Input: part model. Units: mm. Frame: model coordinates. Face numbers are marked on the shaded views. Coordinates: 2 decimals unless noted, no trailing zeros. Loops run counter-clockwise (first coordinate to the right, second up) from the corner with the lowest first, then second, coordinate; pieces in that order, holes last. Notation, with made-up numbers: (-1, -3) - (14, -3) arc R21 ccw to (14, 2) - close; hole circle Ø7 at (-7, -2.75). An arc over 180 degrees is marked (long way). Use a Markdown table: item, result. Add a question column.
1. Section query A-A on y = 0. Return the cut outline in (x, z).
2. Section query B-B on z = 12. Return the cut outline in (x, y), then the cut area to 3 significant figures.
3. Ray query, L1, parallel to X at y = 0, z = 1.2; L2, parallel to X at y = 2.75, z = 4.75. Return the intervals inside material, ascending. Write a range as [from, to].
4. Draft query along Z for the marked faces 1, 2, 3 and 4. Return one class per face: released by +Z, released by -Z, zero draft, split by the parting line, or undercut.
5. Section query D-D on x = 1. Return the cut outline in (y, z), then the cut area to 3 significant figures.
6. Section query C-C on y = 5.25. Return the cut outline in (x, z), then the cut area to 3 significant figures.
7. Contact query for flat-ended pins moving along their axis: P1, Ø5, axis at y = 0, z = 12, coming from the +X side; P2, Ø5.5, axis at y = 0, z = 10.46, coming from the -X side; P3, Ø3.5, axis at x = 9, y = -1.5, coming from the +Z side; P4, Ø2, axis at x = 11.5, z = 3, coming from the -Y side. Output: stop coordinate, or through.
```python
from build123d import *

# Parameters (mm, degrees)
PAD_DEPTH       = 6.35
SKETCH001_R     = 1.778
POCKET_DEPTH    = 14.2758
SKETCH002_R     = 1.778
POCKET001_DEPTH = 14.2758


with BuildPart() as part:
    # Sketch → Pad (new body, symmetric)
    with BuildSketch(Plane.XZ):
        with BuildLine():
            Line((0, 14.2748), (0, 1.27))
            ThreePointArc((0, 1.27), (0.371974, 0.371974), (1.27, 0))
            Line((1.27, 0), (14.2748, 0))
            Line((14.2748, 0), (14.2748, 1.5748))
            Line((14.2748, 1.5748), (2.8448, 1.5748))
            ThreePointArc((1.5748, 2.8448), (1.946774, 1.946774), (2.8448, 1.5748))
            Line((1.5748, 2.8448), (1.5748, 14.2748))
            Line((1.5748, 14.2748), (0, 14.2748))
        make_face()
    extrude(amount=PAD_DEPTH, both=True)

    # Sketch001 → Pocket (cut, through all)
    with BuildSketch(Plane.XY):
        with Locations((10.4648, 0)):
            Circle(SKETCH001_R)
    extrude(amount=POCKET_DEPTH, mode=Mode.SUBTRACT)

    # Sketch002 → Pocket001 (cut, through all)
    with BuildSketch(Plane.YZ):
        with Locations((0, 10.4648)):
            Circle(SKETCH002_R)
    extrude(amount=POCKET001_DEPTH, mode=Mode.SUBTRACT)


solid = part.part
```
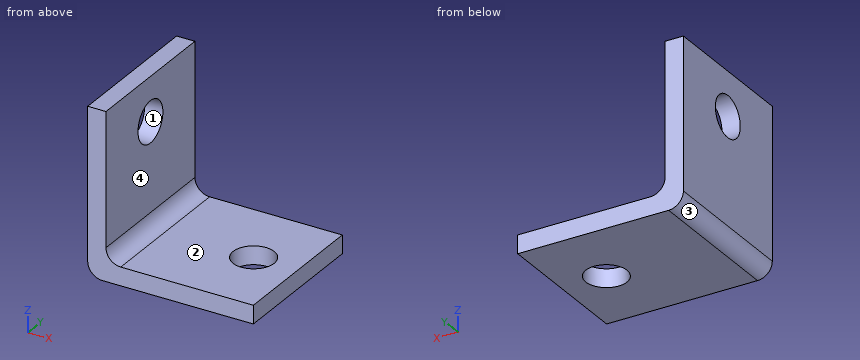
Resolved:
| question | item | result |
|---|---|---|
| 1 | outline | (0, 1.27) arc R1.27 ccw to (1.27, 0) - (8.69, 0) - (8.69, 1.57) - (2.84, 1.57) arc R1.27 cw to (1.57, 2.84) - (1.57, 8.69) - (0, 8.69) - close; (0, 12.24) - (1.57, 12.24) - (1.57, 14.27) - (0, 14.27) - close; (12.24, 0) - (14.27, 0) - (14.27, 1.57) - (12.24, 1.57) - close |
| 2 | outline | (0, -6.35) - (1.57, -6.35) - (1.57, -0.9) - (0, -0.9) - close; (0, 0.9) - (1.57, 0.9) - (1.57, 6.35) - (0, 6.35) - close |
| 2 | area | 17.2 mm² |
| 3 | L1 | [0, 8.69], [12.24, 14.27] |
| 3 | L2 | [0, 1.57] |
| 4 | face 1 | undercut |
| 4 | face 2 | released by +Z |
| 4 | face 3 | released by -Z |
| 4 | face 4 | zero draft |
| 5 | outline | (-6.35, 0.03) - (6.35, 0.03) - (6.35, 14.27) - (-6.35, 14.27) - close; hole circle Ø3.56 at (0, 10.46) |
| 5 | area | 171 mm² |
| 6 | outline | (0, 1.27) arc R1.27 ccw to (1.27, 0) - (14.27, 0) - (14.27, 1.57) - (2.84, 1.57) arc R1.27 cw to (1.57, 2.84) - (1.57, 14.27) - (0, 14.27) - close |
| 6 | area | 42.5 mm² |
| 7 | P1 | x = 1.57 |
| 7 | P2 | x = 0 |
| 7 | P3 | z = 1.57 |
| 7 | P4 | through |
